Can you work these out from the drawing? Everything is in mm from the part's minimum corner. Give positions to 0.01 mm unless a question says otherwise; leave off trailing zeros. Order: outer loops, then holes, each group sorted by start corner. A loop starts at its lowest first (then second) coordinate and runs counter-clockwise, first axis right, second up. Notation, with made-up numbers: (42.5, 42.5) -> (78.5, 42.5) arc R21 cw to (78.5, 46.5) -> close; hole circle Ø8 at (55, 22). An arc over 180 degrees is marked (long way). One line per item, written item: value.
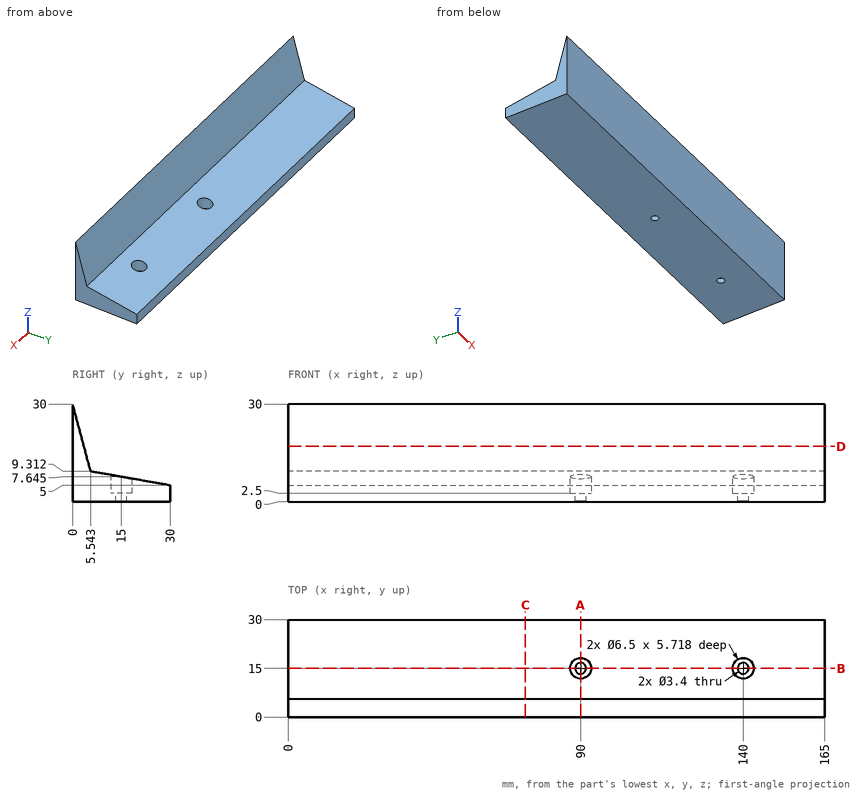
1) Suppose I cut it at B-B, the plane y = 15. State how many separate pieces and enclosed holes the cut face has, then the cut area to 3 significant figures.
Answer below:
separate pieces: 3
enclosed holes: 0
area: 1,180 mm2
2) Suppose I cut it at C-C, the plane x = 73. Write out the boundary of the cut face in (y, z), then the cut area to 3 significant figures.
Answer below:
outline: (0, 0) -> (30, 0) -> (30, 5) -> (5.54, 9.31) -> (0, 30) -> close
area: 284 mm2
3) Suppose I cut it at A-A, the plane x = 90. Write out the boundary of the cut face in (y, z).
Answer below:
outline: (0, 0) -> (13.3, 0) -> (13.3, 2.5) -> (11.75, 2.5) -> (11.75, 8.22) -> (5.54, 9.31) -> (0, 30) -> close; (16.7, 0) -> (30, 0) -> (30, 5) -> (18.25, 7.07) -> (18.25, 2.5) -> (16.7, 2.5) -> close
4) Suppose I cut it at D-D, the plane z = 17. Write out the boundary of the cut face in (x, y).
Answer below:
outline: (0, 0) -> (165, 0) -> (165, 3.48) -> (0, 3.48) -> close
5) If I drill on line 1 along X through (y, z) = (15, 6.8); line 2 along Y through (x, z) = (140, 0.5); line 3 along Y through (x, z) = (90, 4.4), over which ranges is the centre line in solid material (lowest first)?
Answer below:
line 1: x = 0 to 86.75, 93.25 to 136.75, 143.25 to 165
line 2: y = 0 to 13.3, 16.7 to 30
line 3: y = 0 to 11.75, 18.25 to 30
6) For P1, Ø7, axis at x = 90, y = 15, coming from the +Z side; P2, Ø5, axis at x = 90, y = 15, coming from the +Z side; P3, Ø4, axis at x = 28.5, y = 26.5, coming from the +Z side, each with a flat end and sliding along its axis, tell me the tip position at first contact or that it passes through.
Answer below:
P1: stops at z = 8.26
P2: stops at z = 2.5
P3: stops at z = 5.97
